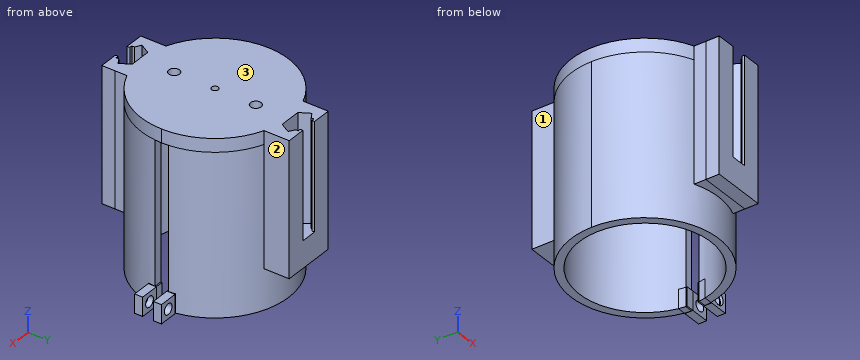
from build123d import *
from build123d.topology import SkipClean

# Parameters (mm, degrees)
SKETCH1_R                       = 34.925
SKETCH1_R_2                     = 15.24
SKETCH1_R_3                     = 2.54
BOSS_EXTRUDE1_DEPTH             = 6.35
BOSS_EXTRUDE2_DEPTH             = 6.35
BOSS_EXTRUDE2_DEPTH_BACK        = 3.81
SKETCH1_2_R                     = 15.24
SKETCH3_R                       = 1.5875
CUT_EXTRUDE2_DEPTH              = 51.425557508
BOSS_EXTRUDE3_START             = 76.2
SKETCH4_R                       = 34.925
SKETCH4_R_2                     = 31.115
BOSS_EXTRUDE3_DEPTH             = 76.2
CUT_EXTRUDE3_START              = 30.48
SKETCH5_W                       = 76.2
SKETCH5_H                       = 6.35
CUT_EXTRUDE3_DEPTH              = 61.327220253
BOSS_EXTRUDE4_START             = 2.54
SKETCH6_W                       = 8.89
SKETCH6_H                       = 8.89
SKETCH6_R                       = 2.5
BOSS_EXTRUDE4_DEPTH             = 3.81
BOSS_EXTRUDE5_START             = -2.54
SKETCH6_2_W                     = 8.89
SKETCH6_2_H                     = 8.89
SKETCH6_2_R                     = 2.5
BOSS_EXTRUDE5_DEPTH             = 3.81
BOSS_EXTRUDE6_REACH             = 111.019
BOSS_EXTRUDE6_END_RADIUS        = 31.115
SKETCH8_W                       = 8.89
SKETCH8_H                       = 3.81
SKETCH9_R                       = 3
SKETCH9_R_2                     = 2.5
CUT_EXTRUDE4_DEPTH              = 1.27
BOSS_EXTRUDE7_REACH             = 116.22
SKETCH12_W                      = 25.4
SKETCH12_H                      = 63.5
BOSS_EXTRUDE7_DIRECTION_2_DEPTH = 6.35
CUT_EXTRUDE5_DEPTH              = 50.8


with BuildPart() as part:
    # Sketch1 → Boss-Extrude1 (new body)
    with BuildSketch(Plane.XY):
        Circle(SKETCH1_R)
        Circle(SKETCH1_R_2, mode=Mode.SUBTRACT)
        with Locations((0, 19.3675)):
            Circle(SKETCH1_R_3, mode=Mode.SUBTRACT)
        with Locations((0, -19.3675)):
            Circle(SKETCH1_R_3, mode=Mode.SUBTRACT)
    extrude(amount=BOSS_EXTRUDE1_DEPTH)

    # Sketch1<2> → Boss-Extrude2 (add, two sides: drawn at the far end of the back side and taken through both)
    with BuildSketch(Plane.XY.offset(-BOSS_EXTRUDE2_DEPTH_BACK)):
        Circle(SKETCH1_2_R)
    extrude(amount=BOSS_EXTRUDE2_DEPTH + BOSS_EXTRUDE2_DEPTH_BACK)

    # Sketch3 → Cut-Extrude2 (cut, through all)
    with BuildSketch(Plane.XY.offset(6.35)):
        Circle(SKETCH3_R)
    extrude(amount=-CUT_EXTRUDE2_DEPTH, mode=Mode.SUBTRACT)

    # Sketch4 → Boss-Extrude3 (add)
    with BuildSketch(Plane(origin=(0, 0, 0), x_dir=(-1, 0, 0), z_dir=(0, 0, -1)).offset(BOSS_EXTRUDE3_START)):
        Circle(SKETCH4_R)
        with Locations(Location((0, 0, 0), (0, 0, 180))):
            Circle(SKETCH4_R_2, mode=Mode.SUBTRACT)
    extrude(amount=-BOSS_EXTRUDE3_DEPTH)

    # Sketch5 → Cut-Extrude3 (cut, through all)
    with SkipClean():  # the faces are left unmerged after this step: merging them gives an invalid solid
        with BuildSketch(Plane(origin=(0, 0, 0), x_dir=(0, 0, -1), z_dir=(1, 0, 0)).offset(CUT_EXTRUDE3_START)):
            with Locations((38.1, 0)):
                Rectangle(SKETCH5_W, SKETCH5_H)
        extrude(amount=CUT_EXTRUDE3_DEPTH, mode=Mode.SUBTRACT)



with BuildPart() as body_2:
    # Sketch6 → Boss-Extrude4 (new body)
    with BuildSketch(Plane(origin=(0, 0, 0), x_dir=(1, 0, 0), z_dir=(0, 1, 0)).offset(BOSS_EXTRUDE4_START)):
        with Locations((39.225382402, 71.755)):
            Rectangle(SKETCH6_W, SKETCH6_H)
        with Locations(Location((39.225382402, 71.755, 0), (0, 0, 90))):
            Circle(SKETCH6_R, mode=Mode.SUBTRACT)
    extrude(amount=BOSS_EXTRUDE4_DEPTH)


with BuildPart() as body_3:
    # Sketch6<2> → Boss-Extrude5 (new body)
    with BuildSketch(Plane(origin=(0, 0, 0), x_dir=(1, 0, 0), z_dir=(0, 1, 0)).offset(BOSS_EXTRUDE5_START)):
        with Locations((39.225382402, 71.755)):
            Rectangle(SKETCH6_2_W, SKETCH6_2_H)
        with Locations(Location((39.225382402, 71.755, 0), (0, 0, 270))):
            Circle(SKETCH6_2_R, mode=Mode.SUBTRACT)
    extrude(amount=-BOSS_EXTRUDE5_DEPTH)


with BuildPart() as part_1:
    with SkipClean():  # the faces are left unmerged after this step: merging them gives an invalid solid
        add(part.part)

        add(body_2.part)  # Boss-Extrude6 merges body 2

        add(body_3.part)  # Boss-Extrude6 merges body 3
        # Boss-Extrude6: up to this cylinder (the profile starts outside it)
        boss_extrude6_end = Plane(origin=(0, 0, -71.755), z_dir=(0, 0, 1)) * Cylinder(BOSS_EXTRUDE6_END_RADIUS, 285.268, mode=Mode.PRIVATE)
        # Sketch8 → Boss-Extrude6 (add, up to the surface)
        with BuildSketch(Plane.ZY.offset(-34.780382402), mode=Mode.PRIVATE) as boss_extrude6_sk1:
            with Locations((-71.755, -4.445)):
                Rectangle(SKETCH8_W, SKETCH8_H)
        boss_extrude6_tool1 = extrude(boss_extrude6_sk1.sketch, amount=BOSS_EXTRUDE6_REACH, mode=Mode.PRIVATE) - boss_extrude6_end
        add(boss_extrude6_tool1.solids().sort_by_distance((34.780382, -4.445, -71.755))[0])
        # Sketch8 → Boss-Extrude6 (add, up to the surface)
        with BuildSketch(Plane.ZY.offset(-34.780382402), mode=Mode.PRIVATE) as boss_extrude6_sk2:
            with Locations((-71.755, 4.445)):
                Rectangle(SKETCH8_W, SKETCH8_H)
        boss_extrude6_tool2 = extrude(boss_extrude6_sk2.sketch, amount=BOSS_EXTRUDE6_REACH, mode=Mode.PRIVATE) - boss_extrude6_end
        add(boss_extrude6_tool2.solids().sort_by_distance((34.780382, 4.445, -71.755))[0])

    # Sketch9 → Cut-Extrude4 (cut)
    with SkipClean():  # the faces are left unmerged after this step: merging them gives an invalid solid
        with BuildSketch(Plane.XZ.offset(6.35)):
            with Locations(Location((39.225382402, -71.755, 0), (0, 0, 270))):
                Circle(SKETCH9_R)
            with Locations(Location((39.225382402, -71.755, 0), (0, 0, 90))):
                Circle(SKETCH9_R_2, mode=Mode.SUBTRACT)
        extrude(amount=-CUT_EXTRUDE4_DEPTH, mode=Mode.SUBTRACT)

    # Sketch12 → Boss-Extrude7 (add, up to next)
    with BuildSketch(Plane(origin=(0, -38.1, 0), x_dir=(1, 0, 0), z_dir=(0, 1, 0)), mode=Mode.PRIVATE) as boss_extrude7_sk1:
        with Locations((0, 25.4)):
            Rectangle(SKETCH12_W, SKETCH12_H)
    boss_extrude7_tool1 = extrude(boss_extrude7_sk1.sketch, amount=BOSS_EXTRUDE7_REACH, mode=Mode.PRIVATE) - part_1.part
    boss_extrude7 = boss_extrude7_tool1.solids().sort_by_distance((0, -38.1, -25.4))[0]
    add(boss_extrude7)

    # Sketch12 → Boss-Extrude7 direction 2 (add)
    with SkipClean():  # the faces are left unmerged after this step: merging them gives an invalid solid
        with BuildSketch(Plane(origin=(0, -38.1, 0), x_dir=(1, 0, 0), z_dir=(0, 1, 0))):
            with Locations((0, 25.4)):
                Rectangle(SKETCH12_W, SKETCH12_H)
        boss_extrude7_direction_2 = extrude(amount=-BOSS_EXTRUDE7_DIRECTION_2_DEPTH)

    # Sketch13 → Cut-Extrude5 (cut)
    with SkipClean():  # the faces are left unmerged after this step: merging them gives an invalid solid
        with BuildSketch(Plane.XY.offset(6.35)):
            Polygon((-3.81, -43.18), (-3.81, -44.45), (3.81, -44.45), (3.81, -43.18), (5.08, -43.18), (5.08, -41.91), (7.829630657, -40.3225), (5.08, -35.56), (-5.08, -35.56), (-7.829630657, -40.3225), (-5.08, -41.91), (-5.08, -43.18), align=None)
        cut_extrude5 = extrude(amount=-CUT_EXTRUDE5_DEPTH, mode=Mode.SUBTRACT)

    # Mirror1: Boss-Extrude7, Boss-Extrude7 direction 2, Cut-Extrude5 across plane
    with SkipClean():  # the faces are left unmerged after this step: merging them gives an invalid solid
        add(boss_extrude7.mirror(Plane.ZX))
        add(boss_extrude7_direction_2.mirror(Plane.ZX))
        add(cut_extrude5.mirror(Plane.ZX), mode=Mode.SUBTRACT)


solid = part_1.part
For this review, take the finished solid that the model builds, in its own axes (mm). Face numbers are marked on the shaded views. A direction names the side the tool comes from. Round coordinates to 2 decimals unless told otherwise and drop trailing zeros. Loops run counter-clockwise (first coordinate to the right, second up) from the corner with the lowest first, then second, coordinate; pieces in that order, holes last. Notation, with made-up numbers: (2, -36.5) - (20, -36.5) arc R23 cw to (20, -4.5) - close; hole circle Ø6 at (54.5, 77.5). An arc over 180 degrees is marked (long way). One line per question, with ' | ' between items.
Q1. Take a section at B-B (z = -71). Give the boundary of the cut face in (x, y) (3 decimals).
Taken from the geometry:
outline: (31.011, -2.54) arc R31.115 cw (long way) to (31.011, 2.54) - (36.842, 2.54) - (36.842, 6.35) - (34.343, 6.35) arc R34.925 ccw (long way) to (34.343, -6.35) - (36.322, -6.35) - (36.322, -5.08) - (36.842, -5.08) - (36.842, -2.54) - close; (41.609, -5.08) - (42.129, -5.08) - (42.129, -6.35) - (43.67, -6.35) - (43.67, -2.54) - (41.609, -2.54) - close; (41.609, 2.54) - (43.67, 2.54) - (43.67, 6.35) - (41.609, 6.35) - close
Q2. Tool access review of the marked faces 1, 2 and 3: name each direction out of +Z, -Z, +X, -X, +Y, -Y from which nothing blocks a thin tool from reaching the whole face with its end or side.
Taken from the geometry:
face 1: +Z, -Z, -X, +Y | face 2: +Z, -Z, +X, +Y | face 3: +Z, +X, -X, +Y, -Y
Q3. Take a section at C-C (y = -27). Give the boundary of the cut face in (x, z).
Taken from the geometry:
outline: (-22.15, -76.2) - (-15.46, -76.2) - (-15.46, 0) - (15.46, 0) - (15.46, -76.2) - (22.15, -76.2) - (22.15, 6.35) - (-22.15, 6.35) - close
Q4. For pin 1 (10 mm diameter, centred on x = 26, z = -59, fed in from +Y); pin 2 (6.5 mm diameter, centred on x = 38.5, z = -73, fed in from -Y); pin 3 (1.5 mm diameter, centred on y = 28, z = -67.5, fed in from +X); pin 4 (8 mm diameter, centred on x = 28, y = 30.5, fed in from +Z), all flat-tipped, find the tip position at first contact; note any pin that passes through.
Taken from the geometry:
pin 1: stops at y = 27.91 | pin 2: stops at y = -6.35 | pin 3: stops at x = 21.84 | pin 4: passes through
Q5. Take a section at D-D (x = 21). Give the boundary of the cut face in (y, z), and give its area (3 significant figures).
Taken from the geometry:
outline: (-27.91, -76.2) - (-22.96, -76.2) - (-22.96, 0) - (22.96, 0) - (22.96, -76.2) - (27.91, -76.2) - (27.91, 6.35) - (-27.91, 6.35) - close | area: 1,110 mm²
Q6. For line 1 along Y through (x, z) = (-4, -32); line 2 along Y through (x, z) = (0, 2); line 3 along Y through (x, z) = (-6, 2), list the stretches that pass through material, from the lowest coordinate up. Write a range as [from, to].
Taken from the geometry:
line 1: y = [-44.45, -43.18], [-35.56, -30.86], [30.86, 35.56], [43.18, 44.45] | line 2: y = [-35.56, -21.91], [-16.83, -1.59], [1.59, 16.83], [21.91, 35.56] | line 3: y = [-44.45, -41.38], [-37.15, 37.15], [41.38, 44.45]
Q7. Take a section at A-A (x = 0). State how many separate pieces and enclosed holes the cut face has, and give its area (3 significant figures).
Taken from the geometry:
separate pieces: 4 | enclosed holes: 0 | area: 1,350 mm²
